CAD build for the part. Positions are in the model's coordinates, mm. Give positions to 0.01 mm unless a question says otherwise; leave off trailing zeros. Order: outer loops, then holes, each group sorted by start corner. A loop starts at its lowest first (then second) coordinate and runs counter-clockwise, first axis right, second up.
```python
from build123d import *

# Parameters (mm, degrees)
PAD_DEPTH     = 3.5
SKETCH001_R   = 2.8
SKETCH001_R_2 = 20
SKETCH001_R_3 = 19.975063
POCKET_DEPTH  = 3.501


with BuildPart() as part:
    # Sketch → Pad (new body)
    with BuildSketch(Plane.XY):
        Polygon((0, 0), (40, 0), (40, 20), (20, 40), (0, 40), (-20, 20), (-20, 0), align=None)
    extrude(amount=PAD_DEPTH)

    # Sketch001 → Pocket (cut, through all)
    with BuildSketch(Plane.XY.offset(3.5)):
        with Locations((10, 30)):
            Circle(SKETCH001_R)
        with Locations((10, 9)):
            Circle(SKETCH001_R)
        with Locations((30, 9)):
            Circle(SKETCH001_R)
        with Locations((-10, 9)):
            Circle(SKETCH001_R)
        with Locations((-20, 40)):
            Circle(SKETCH001_R_2)
        with Locations((40, 40)):
            Circle(SKETCH001_R_3)
    extrude(amount=-POCKET_DEPTH, mode=Mode.SUBTRACT)


solid = part.part
```
Item 1: Two-plate mould, pull along Y, no slides. Class faces 1 (the face through (-7.33, 9.84, 1.77)), 2 (the face through (10, 40, 2)), 3 (the face through (40, 10, 2)): released by +Y, released by -Y, zero draft, split by the parting line, or undercut.
Item 2: Slice it at B-B (z = 0.95). State how many separate pieces and enclosed holes the cut face has, and give its area (3 significant figures).
Item 3: Slice it at D-D (x = 30). Give the cut face in (y, z).
Item 4: Slice it at C-C (x = 10). Give the cut face in (y, z), and give its area (3 significant figures).
Item 5: Slice it at A-A (y = 9). Give the cut face in (x, z).
Item 6: Wall check: L1, parallel to Y at x = 10, z = 0.95; L2, parallel to X at y = 7, z = 1.35; L3, parallel to X at y = 8.5, z = 1 (3 decimals). Give the ranges that are in metal, low to high.
Item 7: Drop flat-ended pins along their axis: pin 1 Ø2 at (x, z) = (-11, 3) entering from +Y; pin 2 Ø2 at (x, z) = (-8, 1) entering from +Y; pin 3 Ø2 at (x, z) = (34, 2.5) entering from +Y; pin 4 Ø9 at (x, y) = (10, 9) entering from +Z. Give the stop position or say it passes through.
A:
1. face 1: undercut
1. face 2: released by +Y
1. face 3: zero draft
2. separate pieces: 1
2. enclosed holes: 4
2. area: 1,670 mm2
3. outline: (0, 0) - (6.2, 0) - (6.2, 3.5) - (0, 3.5) - close; (11.8, 0) - (22.71, 0) - (22.71, 3.5) - (11.8, 3.5) - close
4. outline: (0, 0) - (6.2, 0) - (6.2, 3.5) - (0, 3.5) - close; (11.8, 0) - (27.2, 0) - (27.2, 3.5) - (11.8, 3.5) - close; (32.8, 0) - (40, 0) - (40, 3.5) - (32.8, 3.5) - close
4. area: 101 mm2
5. outline: (-20, 0) - (-12.8, 0) - (-12.8, 3.5) - (-20, 3.5) - close; (-7.2, 0) - (7.2, 0) - (7.2, 3.5) - (-7.2, 3.5) - close; (12.8, 0) - (27.2, 0) - (27.2, 3.5) - (12.8, 3.5) - close; (32.8, 0) - (40, 0) - (40, 3.5) - (32.8, 3.5) - close
6. L1: y = 0 to 6.2, 11.8 to 27.2, 32.8 to 40
6. L2: x = -20 to -11.96, -8.04 to 8.04, 11.96 to 28.04, 31.96 to 40
6. L3: x = -20 to -12.755, -7.245 to 7.245, 12.755 to 27.245, 32.755 to 40
7. pin 1: stops at y = 22.68
7. pin 2: stops at y = 24.8
7. pin 3: stops at y = 21.29
7. pin 4: stops at z = 3.5
